Answer from the drawing. Dimensions are ordinates in mm from the lowest x, y and z of the part. A direction names the side the tool comes from. Coordinates: 2 decimals unless noted, no trailing zeros. Order: outer loops, then holes, each group sorted by start corner. A loop starts at its lowest first (then second) coordinate and runs counter-clockwise, first axis right, second up. Notation, with made-up numbers: (-26.5, 65.25) -> (-4.5, 65.25) arc R13 ccw to (-4.5, 83.25) -> close; hole circle Ø8 at (41.25, 14.5). An arc over 180 degrees is marked (long way). Answer in a Markdown table with one row per item.
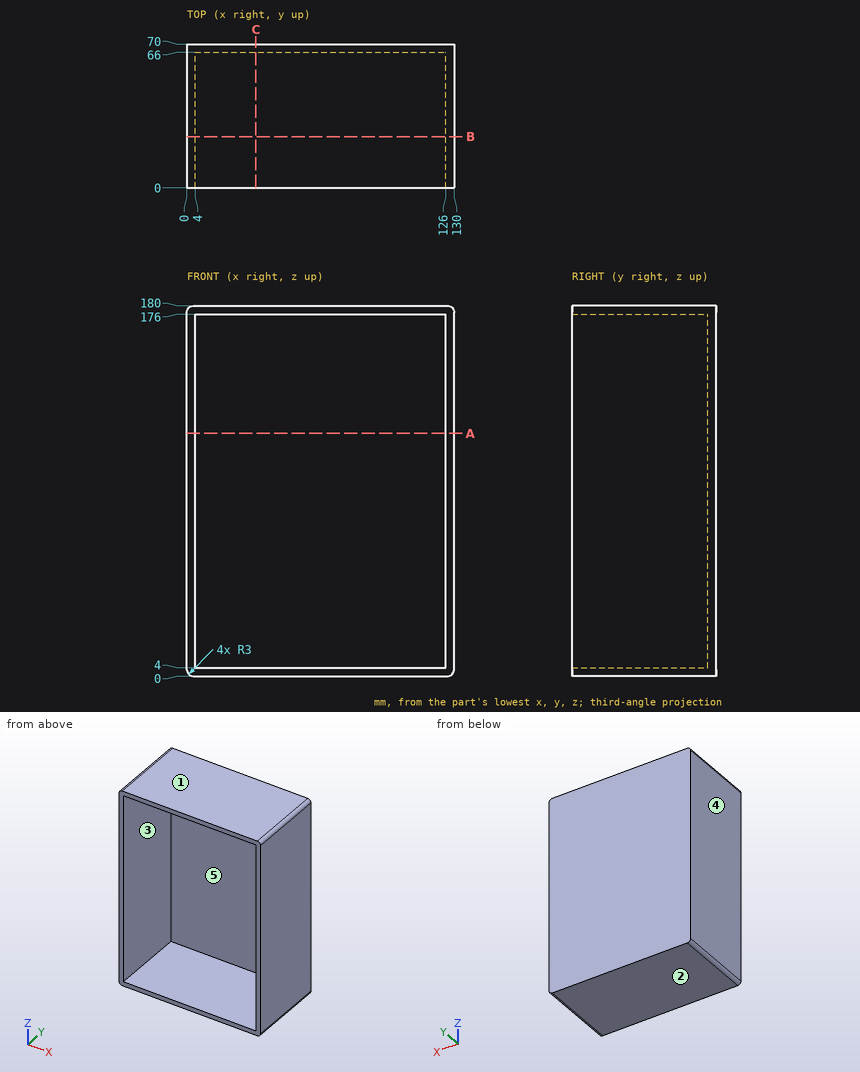
(1) A flat-ended cylindrical pin translates along its axis: pin 1 (12 mm diameter, centred on x = 53.5, z = 158.5, fed in from -Y). Find the tip coordinate at first contact, or state that the pin passes through.
Check values:
| item | result |
|---|---|
| pin 1 | y = 66 |
(2) Which of the six approach directions +Z, -Z, +X, -X, +Y, -Y give full straight-line access (tool end or side, diameter ignored) to the marked faces 4 and 5?
Check values:
| item | result |
|---|---|
| face 4 | +Z, -Z, -X, +Y, -Y |
| face 5 | -Y |
(3) A cutting plane is placed at C-C, the plane x = 33.5. Determine the outline of the cut face in (y, z).
Check values:
| item | result |
|---|---|
| outline | (0, 0) -> (70, 0) -> (70, 180) -> (0, 180) -> (0, 176) -> (66, 176) -> (66, 4) -> (0, 4) -> close |
(4) A cutting plane is placed at B-B, the plane y = 25. Determine the outline of the cut face in (x, z).
Check values:
| item | result |
|---|---|
| outline | (0, 3) arc R3 ccw to (3, 0) -> (127, 0) arc R3 ccw to (130, 3) -> (130, 177) arc R3 ccw to (127, 180) -> (3, 180) arc R3 ccw to (0, 177) -> close; hole (4, 4) -> (126, 4) -> (126, 176) -> (4, 176) -> close |
(5) Find the intervals of material crossed by line 1 along X through (y, z) = (36, 95); line 2 along Z through (x, y) = (110, 59.5); line 3 along Y through (x, z) = (35, 156), in increasing order. Write a range as from..to.
Check values:
| item | result |
|---|---|
| line 1 | 0..4, 126..130 |
| line 2 | 0..4, 176..180 |
| line 3 | 66..70 |
(6) A cutting plane is placed at A-A, the plane z = 118. Determine the outline of the cut face in (x, y), then the cut area to 3 significant figures.
Check values:
| item | result |
|---|---|
| outline | (0, 0) -> (4, 0) -> (4, 66) -> (126, 66) -> (126, 0) -> (130, 0) -> (130, 70) -> (0, 70) -> close |
| area | 1,050 mm² |
(7) For a pull along Z with two mould halves and no side action, classify the marked faces 1, 2 and 3 as released by +Z, released by -Z, zero draft, split by the parting line, or undercut.
Check values:
| item | result |
|---|---|
| face 1 | released by +Z |
| face 2 | released by -Z |
| face 3 | undercut |
